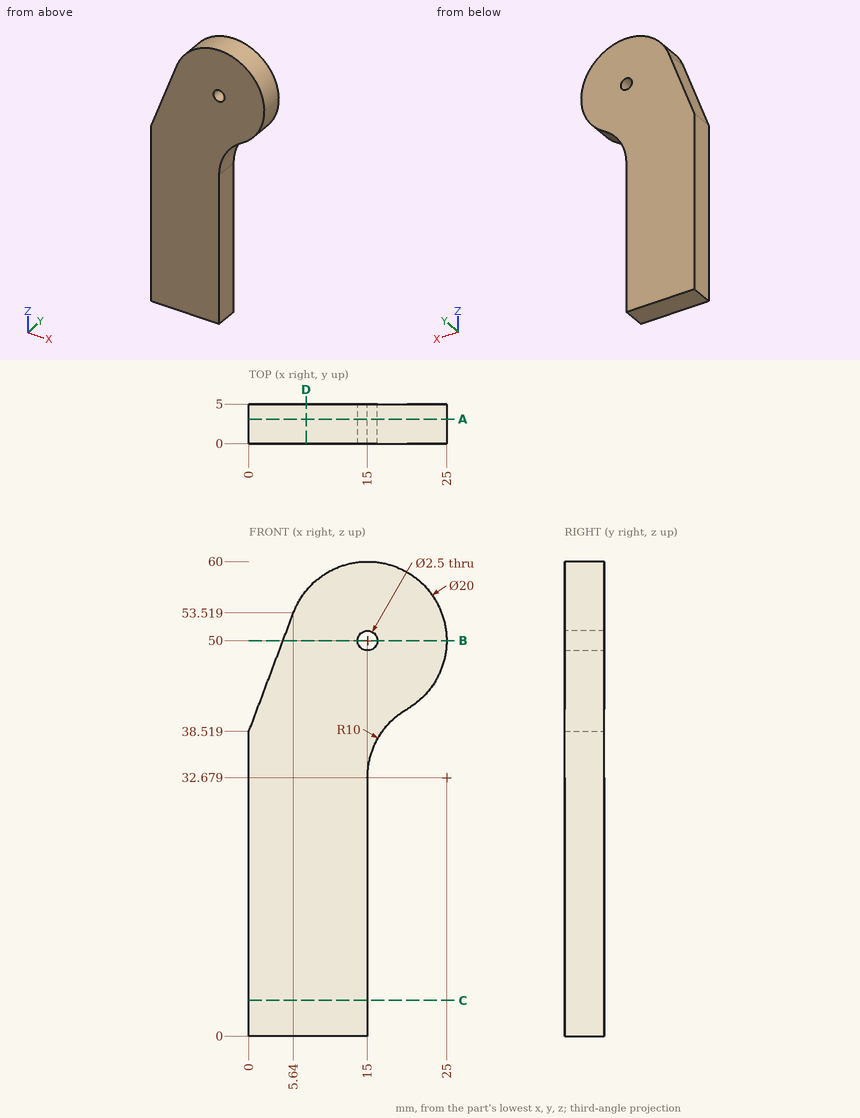
Design review of the part shown in the three views and the two pictorial views. Dimensions are in mm from the part's minimum x, y and z. Round coordinates to 2 decimals unless told otherwise and drop trailing zeros. Write each loop counter-clockwise with the first axis right and the second up, starting at its lowest first coordinate (ties: lowest second). Pieces come first, ordered by that corner, then holes. Notation, with made-up numbers: (75, 75) -> (97, 75) arc R25 ccw to (97, 104) -> close; hole circle Ø6 at (81, 66). An arc over 180 degrees is marked (long way). One line per question, with ' | ' between items. Start each with the question number.
1) For pin 1 Ø3 at (x, z) = (15, 50) entering from +Y; pin 2 Ø1.5 at (x, y) = (5, 2.5) entering from +Z; pin 3 Ø1.5 at (x, y) = (7.5, 2.5) entering from +Z; pin 4 Ø1.5 at (y, z) = (2, 15.5) entering from +X, all flat-tipped, find the tip position at first contact; note any pin that passes through.
2) Wall thickness on line 1 along X through (y, z) = (0.45, 30); line 2 along Z through (x, y) = (9.25, 1.3); line 3 along Z through (x, y) = (9.75, 2.3): over which ranges is each line inside the solid? List them lowest first.
3) Add section B-B (z = 50). Write out the cut boundary in (x, y).
4) Add section D-D (x = 7.25). Write out the cut boundary in (y, z).
5) Add section C-C (z = 4.5). Write out the cut boundary in (x, y), and give its area (3 significant figures).
6) Add section A-A (y = 3.1). Write out the cut boundary in (x, z), and give its area (3 significant figures).
Reported:
1) pin 1: stops at y = 5 | pin 2: stops at z = 53.8 | pin 3: stops at z = 57.38 | pin 4: stops at x = 15
2) line 1: x = 0 to 15 | line 2: z = 0 to 58.18 | line 3: z = 0 to 58.51
3) outline: (4.32, 0) -> (13.75, 0) -> (13.75, 5) -> (4.32, 5) -> close; (16.25, 0) -> (25, 0) -> (25, 5) -> (16.25, 5) -> close
4) outline: (0, 0) -> (5, 0) -> (5, 56.32) -> (0, 56.32) -> close
5) outline: (0, 0) -> (15, 0) -> (15, 5) -> (0, 5) -> close | area: 75.0 mm²
6) outline: (0, 0) -> (15, 0) -> (15, 32.68) arc R10 cw to (20, 41.34) arc R10 ccw (long way) to (5.64, 53.52) -> (0, 38.52) -> close; hole circle Ø2.5 at (15, 50) | area: 965 mm²
